```python
from build123d import *

# Parameters (mm, degrees)
F0_W     = 117.2
F0_H     = 23.39
F1_DEPTH = 3.895
F2_T     = -2.5
F3_DEPTH = 12.5
F4_DEPTH = 12.5


with BuildPart() as f1:
    # F0 (on Front) → F1 (new body, symmetric)
    with BuildSketch(Plane.XZ):
        with Locations((2.3269541562, -20.5496732644)):
            Rectangle(F0_W, F0_H)
    extrude(amount=F1_DEPTH, both=True)

    # F2
    f2_openings = [f1.faces().sort_by_distance(p)[0] for p in [
        (2.326954, -3.895, -20.549673),
    ]]
    offset(amount=F2_T, openings=f2_openings)

    # F3 (cut, symmetric): a face of the model
    f3_faces = [f1.faces().sort_by_distance(p)[0] for p in [
        (60.9269541562, 0, -20.5496732644),
    ]]
    extrude(f3_faces, amount=F3_DEPTH, both=True, mode=Mode.SUBTRACT)

    # F4 (cut, symmetric): a face of the model
    f4_faces = [f1.faces().sort_by_distance(p)[0] for p in [
        (-56.2730458438, 0, -20.5496732644),
    ]]
    extrude(f4_faces, amount=F4_DEPTH, both=True, mode=Mode.SUBTRACT)


solid = f1.part
```
Model file for the job. Use its own axes, mm. A direction names the side the tool comes from. Coordinates: 2 decimals unless noted, no trailing zeros. Write each loop counter-clockwise with the first axis right and the second up, starting at its lowest first coordinate (ties: lowest second). Pieces come first, ordered by that corner, then holes. Notation, with made-up numbers: (-26, 37.25) - (-9, 37.25) arc R30 cw to (-9, 69.25) - close; hole circle Ø5 at (48, -13.75). An arc over 180 degrees is marked (long way). Use a Markdown table: item, result. Add a question column.
Item 1: Band-saw the part on B-B, the plane x = -16. Write the cut outline in (y, z) (3 decimals), and give its area (3 significant figures).
Item 2: Band-saw the part on A-A, the plane y = -0.25. Write the cut outline in (x, z).
Item 3: 3-axis set-ups, long thin cutter, end or side, ignore diameter. For faces 1 (the face through (2, -3.895, -10)), 2 (the face through (2, -1, -11.355)): which of +Z, -Z, +X, -X, +Y, -Y reach the whole face in a straight line?
Item 4: Two-plate mould, pull along Z, no slides. Class faces 3 (the face through (2, 0, -32.245)), 4 (the face through (2, 0, -8.855)), 5 (the face through (2, 1.395, -20)): pulls with the +Z half, pulls with the -Z half, needs draft (parallel to the pull), parting line crosses it, or undercut.
Item 5: Drill centre lines: line 1 along Z through (x, y) = (26.5, 1.25); line 2 along Y through (x, z) = (15, -12.5) (3 decimals). Where is each one in solid material? Low to high.
Item 6: Band-saw the part on C-C, the plane z = -22. Write the cut outline in (x, y) (3 decimals).
Item 7: Drop flat-ended pins along their axis: pin 1 (2 mm diameter, centred on x = 9, z = -15, fed in from -Y) (3 decimals); pin 2 (5 mm diameter, centred on x = -6, z = -29, fed in from -Y) (3 decimals). Give the stop position or say it passes through.
A:
| question | item | result |
|---|---|---|
| 1 | outline | (-3.895, -32.245) - (3.895, -32.245) - (3.895, -8.855) - (-3.895, -8.855) - (-3.895, -11.355) - (1.395, -11.355) - (1.395, -29.745) - (-3.895, -29.745) - close |
| 1 | area | 84.9 mm² |
| 2 | outline | (-43.77, -32.24) - (48.43, -32.24) - (48.43, -29.74) - (-43.77, -29.74) - close; (-43.77, -11.35) - (48.43, -11.35) - (48.43, -8.85) - (-43.77, -8.85) - close |
| 3 | face 1 | +Z, -Z, +X, -X, -Y |
| 3 | face 2 | +X, -X, -Y |
| 4 | face 3 | pulls with the -Z half |
| 4 | face 4 | pulls with the +Z half |
| 4 | face 5 | undercut |
| 5 | line 1 | z = -32.24 to -29.74, -11.35 to -8.85 |
| 5 | line 2 | y = 1.395 to 3.895 |
| 6 | outline | (-43.773, 1.395) - (48.427, 1.395) - (48.427, 3.895) - (-43.773, 3.895) - close |
| 7 | pin 1 | stops at y = 1.395 |
| 7 | pin 2 | stops at y = -3.895 |
